Autodesk Inventor part; units mm, degrees
ref_plane "YZ Plane" through (0, 0, 0) normal (1, 0, 0) x (0, 1, 0)
ref_plane "XZ Plane" through (0, 0, 0) normal (0, 1, 0) x (-1, 0, 0)
ref_plane "XY Plane" through (0, 0, 0) normal (0, 0, 1) x (1, 0, 0)
sketch "Boceto1" plane through (0, 0, 0) normal (1, 0, 0) x (0, 1, 0)
  circle A0 centre (0, 0) radius 2.9
  line L0 (2.2, 1.8894) -> (2.2, -1.8894)
  line L1 (-2.2, 1.8894) -> (-2.2, -1.8894)
  circle A1 centre (0, 0) radius 6.5
  dimension "d0" = 5.8
  dimension "d1" = 2.2
  dimension "d2" = 2.2
  dimension "d3" = 13
extrude "Extrusión1" add sketch "Boceto1" along normal blind 9 contours A0 L0 | L1 A0 | A1
sketch "Boceto2" plane through (9, 0, 0) normal (1, 0, 0) x (0, 0, -1)
  circle A0 centre (0, 0) radius 6.5
  line L0 (3.35, -3.35) -> (-3.35, -3.35)
  line L1 (-3.35, -3.35) -> (-3.35, 3.35)
  line L2 (-3.35, 3.35) -> (3.35, 3.35)
  line L3 (3.35, 3.35) -> (3.35, -3.35)
  line L4 (3.35, -3.35) -> (-3.35, 3.35) construction
  line L5 (-3.35, -3.35) -> (3.35, 3.35) construction
  dimension "d6" = 6.7
  dimension "d7" = 6.7
extrude "Extrusión2" add sketch "Boceto2" along normal blind 10
properties part number "Adaptador"
CAD build for the part. Positions are in the model's coordinates, mm. A direction names the side the tool comes from. Give positions to 0.01 mm unless a question says otherwise; leave off trailing zeros. Loops run counter-clockwise (first coordinate to the right, second up) from the corner with the lowest first, then second, coordinate; pieces in that order, holes last. Notation, with made-up numbers: M 46.5,-15.75 L 78.5,-15.75 A7 ccw 78.5,-2.75 Z; hole C -33,-26.5 d1. An arc over 180 degrees is marked long. Write each question's results on one line, items separated by ' | '.
Q1. Probe probe 1 along Y at (x, z) = (16.25, -1.75); probe 2 along Z at (x, y) = (17.25, -3.25); probe 3 along Z at (x, y) = (9.5, 0.25). List the from-to ranges inside material, lowest first.
Geometry check:
probe 1: y = -6.26 to -3.35, 3.35 to 6.26 | probe 2: z = -5.63 to -3.35, 3.35 to 5.63 | probe 3: z = -6.5 to -3.35, 3.35 to 6.5
Q2. Band-saw the part on A-A on y = -1.25. Write the cut outline in (x, z), and give its area (3 significant figures).
Geometry check:
outline: M 0,-6.38 L 19,-6.38 L 19,-3.35 L 9,-3.35 L 9,-2.62 L 0,-2.62 Z; M 0,2.62 L 9,2.62 L 9,3.35 L 19,3.35 L 19,6.38 L 0,6.38 Z | area: 128 mm²
Q3. Which spindle directions (+Z, -Z, +X, -X, +Y, -Y) get a long thin tool onto all of the face, cutting with end or side? Do faces 1 (the face through (19, 0, -4)), 2 (the face through (14, 0, -3.35)), 3 (the face through (4, 2.2, 0)). Say none if no direction does.
Geometry check:
face 1: +Z, -Z, +X, +Y, -Y | face 2: +X | face 3: +X, -X
Q4. Flat gauge pins, fed straight in: P1, Ø2, axis at x = 16.5, z = 0.5, coming from the +Y side; P2, Ø5, axis at x = 3, y = -5, coming from the -Z side; P3, Ø2, axis at x = 16, z = -4.5, coming from the -Y side; P4, Ø2, axis at x = 16, y = -1.5, coming from the -Z side. Where does each tip first touch, or does it go through?
Geometry check:
P1: stops at y = 6.5 | P2: stops at z = -6 | P3: stops at y = -5.48 | P4: stops at z = -6.48
Q5. Band-saw the part on B-B on x = 11.5. Write the cut outline in (y, z).
Geometry check:
outline: C 0,0 d13; hole M -3.35,-3.35 L 3.35,-3.35 L 3.35,3.35 L -3.35,3.35 Z
Q6. Mould opens along Y. For faces 4 (the face through (4.4, 0, -2.9)), 5 (the face through (0, 3, 0)), 6 (the face through (7.26, 3.07, -5.73)) say: pulls with the +Y half, pulls with the -Y half, needs draft (parallel to the pull), parting line crosses it, or undercut.
Geometry check:
face 4: undercut | face 5: needs draft | face 6: parting line crosses it
